The model under review builds one solid part; all positions refer to its coordinate system, in mm. Face numbers are marked on the shaded views. A direction names the side the tool comes from. Coordinates: 2 decimals unless noted, no trailing zeros. Write each loop counter-clockwise with the first axis right and the second up, starting at its lowest first coordinate (ties: lowest second). Pieces come first, ordered by that corner, then holes. Notation, with made-up numbers: M 27,-3.5 L 59,-3.5 A33 ccw 59,32.5 Z; hole C 23.5,14 d9. An arc over 180 degrees is marked long. Answer as CSV lines item,"result". Start each with the question number.
from build123d import *

# Parameters (mm, degrees)
BOSS_EXTRUDE1_DEPTH     = 44.45
FILLET1_R               = 6.35
FILLET2_R               = 6.35
SKETCH4_R               = 3.96875
CUT_EXTRUDE2_DEPTH      = 254
CUT_EXTRUDE4_DEPTH      = 150.461249158
CUT_EXTRUDE4_DEPTH_BACK = 150.461249158
SKETCH5_W               = 11.43
SKETCH5_H               = 31.75


with BuildPart() as part:
    # Sketch1 → Boss-Extrude1 (new body)
    with BuildSketch(Plane(origin=(0, 0, 0), x_dir=(1, 0, 0), z_dir=(0, 1, 0))):
        Polygon((0, 0), (0, 57.15), (133.35, 57.15), (133.35, 0), (127, 0), (127, 50.8), (6.35, 50.8), (6.35, 0), align=None)
    extrude(amount=BOSS_EXTRUDE1_DEPTH)

    # Fillet1
    fillet1_edges = [part.edges().sort_by_distance(p)[0] for p in [
        (6.35, 22.225, -50.8),
        (127, 22.225, -50.8),
    ]]
    fillet(fillet1_edges, radius=FILLET1_R)

    # Fillet2
    fillet2_edges = [part.edges().sort_by_distance(p)[0] for p in [
        (127, 22.225, 0),
        (6.35, 22.225, 0),
    ]]
    fillet(fillet2_edges, radius=FILLET2_R - 0.0001)  # a hair under: the kernel refuses the full size

    # Sketch4 → Cut-Extrude2 (cut)
    with BuildSketch(Plane(origin=(139.7, 1.415162488, -69.948790088), x_dir=(0, 0, -1), z_dir=(1, 0, 0))):
        with Locations((-54.708790088, 20.809837512)):
            Circle(SKETCH4_R)
    extrude(amount=-CUT_EXTRUDE2_DEPTH, mode=Mode.SUBTRACT)

    # Sketch5 → Cut-Extrude4 (cut, two sides: drawn at the far end of the back side and taken through both)
    with BuildSketch(Plane.XY.offset(-50.8).offset(-CUT_EXTRUDE4_DEPTH_BACK)):
        with Locations((118.745, 22.225)):
            Rectangle(SKETCH5_W, SKETCH5_H)
    extrude(amount=CUT_EXTRUDE4_DEPTH + CUT_EXTRUDE4_DEPTH_BACK, mode=Mode.SUBTRACT)


solid = part.part
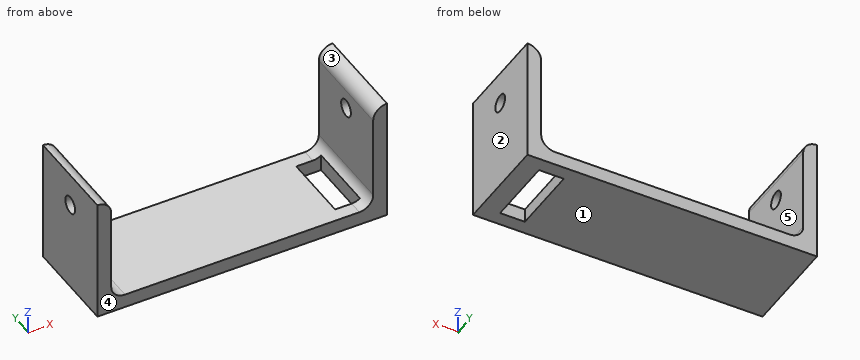
1) Clearance check with flat-ended pins moving along their axes: pin 1 Ø10 at (x, y) = (14.5, 12) entering from +Z; pin 2 Ø6 at (y, z) = (9.5, -30) entering from -X; pin 3 Ø2 at (x, y) = (48.5, 33.5) entering from +Z. State where each tip first meets the part, or that it passes through.
2) To check wall thickness, follow line 1 (X direction, y = 11.5, z = -13); line 2 (Y direction, x = 131, z = -15); line 3 (Z direction, x = 75.5, y = 41.5). State the ranges of each line that lie inside material, in increasing order. Write a range as [from, to].
3) Mouldability with a two-part tool opening along X and no side actions: class the marked faces 1, 2 and 3 as +X half, -X half, draft (parallel to the pull), parting line (faces both ways), or undercut.
4) Take a section at D-D on z = -46.5. Give the boundary of the cut face in (x, y).
5) Take a section at A-A on z = -22. Give the boundary of the cut face in (x, y), and give its area (3 significant figures).
6) Tool access review of the marked faces 4 and 5: name each direction out of +Z, -Z, +X, -X, +Y, -Y from which nothing blocks a thin tool from reaching the whole face with its end or side.
7) Take a section at B-B on z = -15.24. Give the boundary of the cut face in (x, y).
Results:
1,pin 1,"stops at z = -49.93"
1,pin 2,"stops at x = 0"
1,pin 3,"stops at z = -50.8"
2,line 1,"x = [0, 6.35], [127, 133.35]"
2,line 2,"y = [0, 18.26], [26.19, 44.45]"
2,line 3,"z = [-57.15, -50.8]"
3,face 1,"draft"
3,face 2,"+X half"
3,face 3,"undercut"
4,outline,"M 0,0 L 6.69,0 L 6.69,44.45 L 0,44.45 Z; M 126.66,0 L 133.35,0 L 133.35,44.45 L 126.66,44.45 Z"
5,outline,"M 0,0 L 6.35,0 L 6.35,44.45 L 0,44.45 Z; M 127,0 L 133.35,0 L 133.35,44.45 L 127,44.45 Z"
5,area,"565 mm²"
6,face 4,"+Z, -Z, +X, -X, -Y"
6,face 5,"+Z, +Y, -Y"
7,outline,"M 0,0 L 6.35,0 L 6.35,18.26 L 0,18.26 Z; M 0,26.19 L 6.35,26.19 L 6.35,44.45 L 0,44.45 Z; M 127,0 L 133.35,0 L 133.35,18.26 L 127,18.26 Z; M 127,26.19 L 133.35,26.19 L 133.35,44.45 L 127,44.45 Z"
